Source: CAD feature listing. Evaluate the final solid. Frame: model axes, mm. Face numbers are marked on the shaded views. A direction names the side the tool comes from. Give positions to 0.01 mm unless a question says otherwise; leave off trailing zeros. Order: outer loops, then holes, each group sorted by start corner. A loop starts at its lowest first (then second) coordinate and runs counter-clockwise, first axis right, second up.
from build123d import *

# Parameters (mm, degrees)
F3_DEPTH      = 56.0778768191
F3_DEPTH_BACK = 56.0778768191
F5_DEPTH      = 56.0778769191
F5_DEPTH_BACK = 56.0778769191


with BuildPart() as f1:
    # F0 (on Front) → F1 (revolve)
    with BuildSketch(Plane.XZ):
        Polygon((0, -57.1250468493), (-15.5477952212, -57.1250468493), (-11.3551309332, -44.5470511913), (-20.4713844212, -35.7113393235), (-15.8971827477, -22.5355681032), (-26.5535367653, -9.2588011175), (-21.1380142719, 4.3673580512), (-32.4480030819, 16.3774517456), (-28.8245640695, 29.8727303743), (-37.5592783093, 38.6074446142), (-56.0768768191, 38.6074446142), (-56.0768768191, -72.1487551928), (0, -72.1487551928), align=None)
    revolve(axis=Axis((0, 0, -64.636901021), (0, 0, -1)))

    # F2 (on Front) → F3 (cut, two sides)
    with BuildSketch(Plane.XZ) as f3_sk:
        Polygon((-81.2481045723, -62.1343776584), (-79.4872939587, -92.5083234906), (101.4357730746, -92.5083234906), (101.4357730746, -60.3735670447), (12.955147773, -60.3735670447), (12.955147773, 0), (-12.1363736689, 0), (-12.1363736689, -62.1343776584), align=None)
        with BuildLine():
            ThreePointArc((12.955147773, 0), (0.4093870521, 12.545760721), (-12.1363736689, 0))
            Line((-12.1363736689, 0), (12.955147773, 0))
        make_face()
    extrude(amount=-F3_DEPTH, mode=Mode.SUBTRACT)
    extrude(f3_sk.sketch, amount=F3_DEPTH_BACK, mode=Mode.SUBTRACT)

    # F4 (on Right) → F5 (cut, two sides)
    with BuildSketch(Plane.YZ) as f5_sk:
        with BuildLine():
            Line((12.0539087802, -70.0524225831), (12.0539087802, 0))
            ThreePointArc((12.0539087802, 0), (0.1746942289, 11.8792145513), (-11.7045203224, 0))
            Line((-11.7045203224, 0), (-11.7045203224, -70.0524225831))
            Line((-11.7045203224, -70.0524225831), (12.0539087802, -70.0524225831))
        make_face()
    extrude(amount=-F5_DEPTH, mode=Mode.SUBTRACT)
    extrude(f5_sk.sketch, amount=F5_DEPTH_BACK, mode=Mode.SUBTRACT)


solid = f1.part
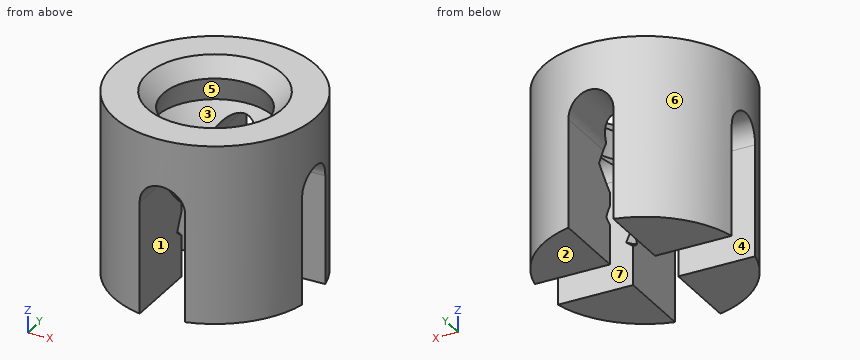
1) Pull-direction query (X, two-part tool) for the marked faces 5, 6 and 7; classes: +X half, -X half, draft (parallel to the pull), parting line (faces both ways), or undercut.
Checks:
face 5: undercut
face 6: parting line
face 7: draft
2) First-contact query: pin 1 Ø3 at (x, y) = (42.5, 20.5) entering from -Z; pin 2 Ø12 at (y, z) = (-37.5, 27.5) entering from -X; pin 3 Ø21.5 at (x, z) = (-27.5, -35) entering from +Y; pin 4 Ø4 at (x, y) = (36, -4) entering from +Z. Flat tips, straight axial feed; report the tip coordinate or a pass-through.
Checks:
pin 1: stops at z = -60.37
pin 2: stops at x = -46.39
pin 3: stops at y = 53.52
pin 4: stops at z = 38.61
3) Ray query, L1, parallel to Z at x = 17, y = -50; L2, parallel to X at y = 19, z = -48.5; L3, parallel to X at y = -42, z = -16. Return the intervals inside material, ascending.
Checks:
L1: z = -60.37 to 38.61
L2: x = -52.76 to -12.14, 12.96 to 52.76
L3: x = -37.16 to -12.14, 12.96 to 37.16
4) Section query B-B on y = 0. Output: boundary loops of the cut face in (x, z), and give its area (3 significant figures).
Checks:
outline: (-56.08, 11.88) - (-28.21, 11.88) - (-32.45, 16.38) - (-28.82, 29.87) - (-37.56, 38.61) - (-56.08, 38.61) - close; (28.21, 11.88) - (56.08, 11.88) - (56.08, 38.61) - (37.56, 38.61) - (28.82, 29.87) - (32.45, 16.38) - close
area: 1,320 mm2
5) Reachability of the marked faces 1, 2, 3 and 4 from +Z, -Z, +X, -X, +Y, -Y: full face, straight path, thin tool, end or side. Return the list, or none.
Checks:
face 1: -Z, +Y, -Y
face 2: -Z, +X, +Y, -Y
face 3: none
face 4: -Z, +X, -X
6) Section query C-C on x = 45. Output: boundary loops of the cut face in (y, z), and give its area (3 significant figures).
Checks:
outline: (-33.46, -60.37) - (-11.7, -60.37) - (-11.7, 0) arc R11.88 cw to (12.05, 0) - (12.05, -60.37) - (33.46, -60.37) - (33.46, 38.61) - (-33.46, 38.61) - close
area: 4,970 mm2
7) Section query A-A on x = 0. Output: boundary loops of the cut face in (y, z).
Checks:
outline: (-56.08, 12.54) - (-28.83, 12.54) - (-32.45, 16.38) - (-28.82, 29.87) - (-37.56, 38.61) - (-56.08, 38.61) - close; (28.82, 29.87) - (32.45, 16.38) - (28.83, 12.54) - (56.08, 12.54) - (56.08, 38.61) - (37.56, 38.61) - close
8) Section query D-D on y = -48.5. Output: boundary loops of the cut face in (x, z).
Checks:
outline: (-28.15, -62.13) - (-12.14, -62.13) - (-12.14, 0) arc R12.55 cw to (12.96, 0) - (12.96, -60.37) - (28.15, -60.37) - (28.15, 38.61) - (-28.15, 38.61) - close
